Job drawing, mm, ordinate dimensions from the low corner. One solid piece. A direction names the side the tool comes from. Round coordinates to 2 decimals unless told otherwise and drop trailing zeros. Loops run counter-clockwise (first coordinate to the right, second up) from the corner with the lowest first, then second, coordinate; pieces in that order, holes last.
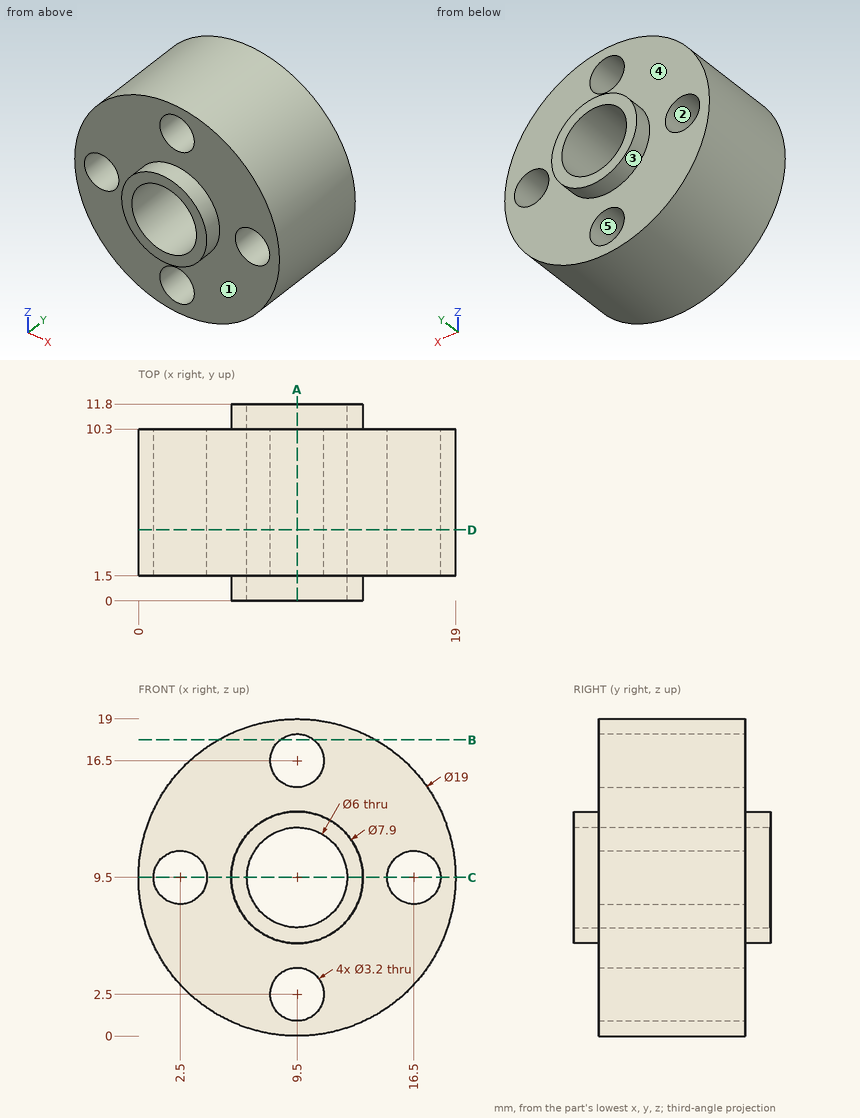
(1) Probe line 1 (X direction, y = 5.25, z = 9.5); line 2 (Y direction, x = 13.75, z = 12.75); line 3 (X direction, y = 4.5, z = 10.5). List the from-to ranges inside material, lowest first.
Responses:
line 1: x = 0 to 0.9, 4.1 to 6.5, 12.5 to 14.9, 18.1 to 19
line 2: y = 1.5 to 10.3
line 3: x = 0.05 to 1.25, 3.75 to 6.67, 12.33 to 15.25, 17.75 to 18.95
(2) Slice it at A-A on x = 9.5. List the corners of the cut face in (y, z), plus the area to 3 significant figures.
Responses:
outline: (0, 5.55) - (1.5, 5.55) - (1.5, 4.1) - (10.3, 4.1) - (10.3, 5.55) - (11.8, 5.55) - (11.8, 6.5) - (0, 6.5) - close; (0, 12.5) - (11.8, 12.5) - (11.8, 13.45) - (10.3, 13.45) - (10.3, 14.9) - (1.5, 14.9) - (1.5, 13.45) - (0, 13.45) - close; (1.5, 0) - (10.3, 0) - (10.3, 0.9) - (1.5, 0.9) - close; (1.5, 18.1) - (10.3, 18.1) - (10.3, 19) - (1.5, 19) - close
area: 63.8 mm2
(3) Pin check, flat tips, straight feed: P1, Ø3.5, axis at x = 2.5, z = 9.5, coming from the +Y side; P2, Ø1.5, axis at y = 3.5, z = 7.5, coming from the -X side; P3, Ø1, axis at x = 8.5, z = 4, coming from the -Y side. Stop position of each tip, or through.
Responses:
P1: stops at y = 10.3
P2: stops at x = 0.08
P3: stops at y = 1.5
(4) Which spindle directions (+Z, -Z, +X, -X, +Y, -Y) get a long thin tool onto all of the face, cutting with end or side? Do the marked faces 1 and 2. Say none if no direction does.
Responses:
face 1: -Y
face 2: +Y, -Y
(5) Slice it at D-D on y = 4.25. List the corners of the cut face in (x, z), plus the area to 3 significant figures.
Responses:
outline: circle Ø19 at (9.5, 9.5); hole circle Ø3.2 at (2.5, 9.5); hole circle Ø6 at (9.5, 9.5); hole circle Ø3.2 at (9.5, 2.5); hole circle Ø3.2 at (9.5, 16.5); hole circle Ø3.2 at (16.5, 9.5)
area: 223 mm2
(6) Pull direction Z, two halves, no side cores. Call the marked faces 3, 4 and 5: +Z half, -Z half, draft (parallel to the pull), parting line (faces both ways), or undercut.
Responses:
face 3: parting line
face 4: draft
face 5: undercut
(7) Slice it at C-C on z = 9.5. List the corners of the cut face in (x, y), plus the area to 3 significant figures.
Responses:
outline: (0, 1.5) - (0.9, 1.5) - (0.9, 10.3) - (0, 10.3) - close; (4.1, 1.5) - (5.55, 1.5) - (5.55, 0) - (6.5, 0) - (6.5, 11.8) - (5.55, 11.8) - (5.55, 10.3) - (4.1, 10.3) - close; (12.5, 0) - (13.45, 0) - (13.45, 1.5) - (14.9, 1.5) - (14.9, 10.3) - (13.45, 10.3) - (13.45, 11.8) - (12.5, 11.8) - close; (18.1, 1.5) - (19, 1.5) - (19, 10.3) - (18.1, 10.3) - close
area: 63.8 mm2
(8) Slice it at B-B on z = 17.75. List the corners of the cut face in (x, y), plus the area to 3 significant figures.
Responses:
outline: (4.79, 1.5) - (8.5, 1.5) - (8.5, 10.3) - (4.79, 10.3) - close; (10.5, 1.5) - (14.21, 1.5) - (14.21, 10.3) - (10.5, 10.3) - close
area: 65.3 mm2
